Check sheet for the modelled part. Datum: model origin and axes. Units: mm. Face numbers are marked on the shaded views. Coordinates: 2 decimals unless noted, no trailing zeros. Order: outer loops, then holes, each group sorted by start corner. A loop starts at its lowest first (then second) coordinate and runs counter-clockwise, first axis right, second up.
from build123d import *

# Parameters (mm, degrees)
CROQUIS1_W              = 41.4
CROQUIS1_H              = 40.4
CROQUIS1_R              = 1.5
SALIENTE_EXTRUIR1_DEPTH = 5
CROQUIS3_W              = 35.2
CROQUIS3_H              = 40.4
CROQUIS3_R              = 1.5
SALIENTE_EXTRUIR3_DEPTH = 5
CORTAR_EXTRUIR1_REACH   = 77.812
REDONDEO1_R             = 20
CORTAR_EXTRUIR2_REACH   = 77.812


with BuildPart() as part:
    # Croquis1 → Saliente-Extruir1 (new body)
    with BuildSketch(Plane.XY):
        with Locations((52.2, 0)):
            Rectangle(CROQUIS1_W, CROQUIS1_H)
        with Locations((63.5, 0)):
            Circle(CROQUIS1_R, mode=Mode.SUBTRACT)
        with Locations((63.5, -15.5)):
            Circle(CROQUIS1_R, mode=Mode.SUBTRACT)
        with Locations((38, 0)):
            Circle(CROQUIS1_R, mode=Mode.SUBTRACT)
        with Locations((63.5, 15.5)):
            Circle(CROQUIS1_R, mode=Mode.SUBTRACT)
        with Locations((67, -7.75)):
            Circle(CROQUIS1_R, mode=Mode.SUBTRACT)
        with Locations((67, 7.75)):
            Circle(CROQUIS1_R, mode=Mode.SUBTRACT)
    extrude(amount=SALIENTE_EXTRUIR1_DEPTH)

    # Croquis3 → Saliente-Extruir3 (add)
    with BuildSketch(Plane.XY.offset(5)):
        with Locations((13.9, 0)):
            Rectangle(CROQUIS3_W, CROQUIS3_H)
        with Locations((8.5, 0)):
            Circle(CROQUIS3_R, mode=Mode.SUBTRACT)
        with Locations((8.5, -10)):
            Circle(CROQUIS3_R, mode=Mode.SUBTRACT)
        with Locations((8.5, 10)):
            Circle(CROQUIS3_R, mode=Mode.SUBTRACT)
        with Locations((12, 8)):
            Circle(CROQUIS3_R, mode=Mode.SUBTRACT)
        with Locations((12, -8)):
            Circle(CROQUIS3_R, mode=Mode.SUBTRACT)
    extrude(amount=-SALIENTE_EXTRUIR3_DEPTH)

    # Croquis5 → Cortar-Extruir1 (cut, up to next)
    with BuildSketch(Plane.XY.offset(5), mode=Mode.PRIVATE) as cortar_extruir1_sk1:
        with BuildLine():
            Line((7.014997686, 20.2), (56.8, 20.2))
            add(Edge.make_bspline(
                [(56.8, 20.2), (28.469554023, 9.322898051), (7.014997686, 20.2)],
                knots=[0, 0, 0, 0.793600416, 0.793600416, 0.793600416], degree=2))
        make_face()
    cortar_extruir1_tool1 = extrude(cortar_extruir1_sk1.sketch, amount=-CORTAR_EXTRUIR1_REACH, mode=Mode.PRIVATE) & part.part
    cortar_extruir1 = cortar_extruir1_tool1.solids().sort_by_distance((31.21991, 18.02458, 5))[0]
    add(cortar_extruir1, mode=Mode.SUBTRACT)

    # Simetría1: Cortar-Extruir1 across plane
    add(cortar_extruir1.mirror(Plane.ZX), mode=Mode.SUBTRACT)

    # Redondeo1
    # the kernel refuses this fillet: 20 mm, written as the material it takes off along each edge
    with BuildSketch(Plane(origin=(-3.7, 20.2, 49.285207182), x_dir=(1, 0, 0), z_dir=(0, 0, -1))) as redondeo1_piece_1:
        with BuildLine():
            CenterArc((20, 17.714082873), REDONDEO1_R, 180, 62.338298383)
            Line((0, 17.714082873), (-0.4, 17.714082873))
            Line((-0.4, 17.714082873), (-0.4, 0))
            Line((-0.4, 0), (0, -0.4))
            ThreePointArc((0, -0.4), (5.357498843, -0.4), (10.52929764, -0.354281657))
            Line((10.52929764, -0.354281657), (10.714997686, 0))
        make_face()
    extrude(amount=93.570414364, mode=Mode.SUBTRACT)

    # Croquis6 → Cortar-Extruir2 (cut, up to next)
    with BuildSketch(Plane.XY.offset(5), mode=Mode.PRIVATE) as cortar_extruir2_sk1:
        with BuildLine():
            ThreePointArc((57.606275, 11.70586502), (57.004955729, 12.658789554), (56.35736085, 13.580890908))
            Line((56.35736085, 13.580890908), (48.977815911, 9.082196509))
            ThreePointArc((48.977815911, 9.082196509), (52.247762477, 0), (48.977815911, -9.082196509))
            Line((48.977815911, -9.082196509), (57.606275, -14.342249927))
            Line((57.606275, -14.342249927), (57.606275, 11.70586502))
        make_face()
    cortar_extruir2_tool1 = extrude(cortar_extruir2_sk1.sketch, amount=-CORTAR_EXTRUIR2_REACH, mode=Mode.PRIVATE) & part.part
    add(cortar_extruir2_tool1.solids().sort_by_distance((54.420947, -0.132696, 5))[0], mode=Mode.SUBTRACT)


solid = part.part
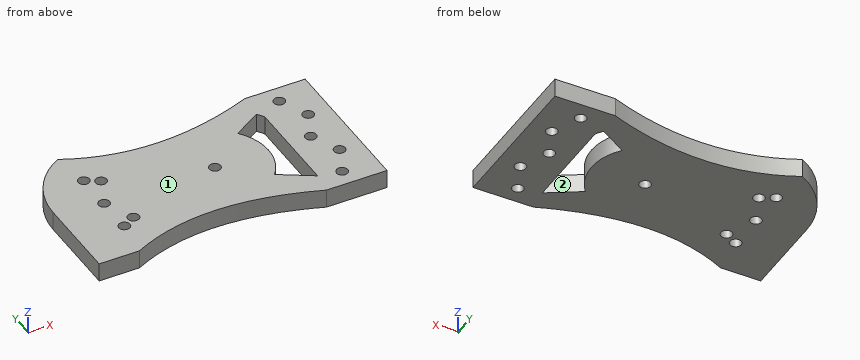
(1) Release check for a two-part mould opening along Y. For the marked faces 1 and 2 record: +Y half, -Y half, draft (parallel to the pull), parting line (faces both ways), or undercut.
Filled in:
face 1: draft
face 2: undercut
(2) Cross-section at A-A (x = 63.5). Enter the section's corners in (y, z), and give its area (3 significant figures).
Filled in:
outline: (-20.2, 0) - (-17, 0) - (-17, 5) - (-20.2, 5) - close; (-14, 0) - (-1.5, 0) - (-1.5, 5) - (-14, 5) - close; (1.5, 0) - (14, 0) - (14, 5) - (1.5, 5) - close; (17, 0) - (20.2, 0) - (20.2, 5) - (17, 5) - close
area: 157 mm2
(3) Go/stop test with a flat-tipped pin: P1, Ø1, axis at x = 26.5, z = 3, coming from the -Y side. Record where the tip stops, or that it passes through.
Filled in:
P1: stops at y = -14.92
(4) Cross-section at B-B (z = 2.85). Count the separate pieces of the cut face and the enclosed holes in it, and give its area (3 significant figures).
Filled in:
separate pieces: 1
enclosed holes: 12
area: 2,440 mm2
(5) Thickness scan on probe 1 along Y at (x, z) = (67, 3.25); probe 2 along Y at (x, z) = (12, 2.4); probe 3 along Y at (x, z) = (63.5, 0.95). Record the ranges inside material, lowest first.
Filled in:
probe 1: y = -20.2 to -9.25, -6.25 to 6.25, 9.25 to 20.2
probe 2: y = -18 to -9.5, -6.5 to 6.5, 9.5 to 18
probe 3: y = -20.2 to -17, -14 to -1.5, 1.5 to 14, 17 to 20.2
